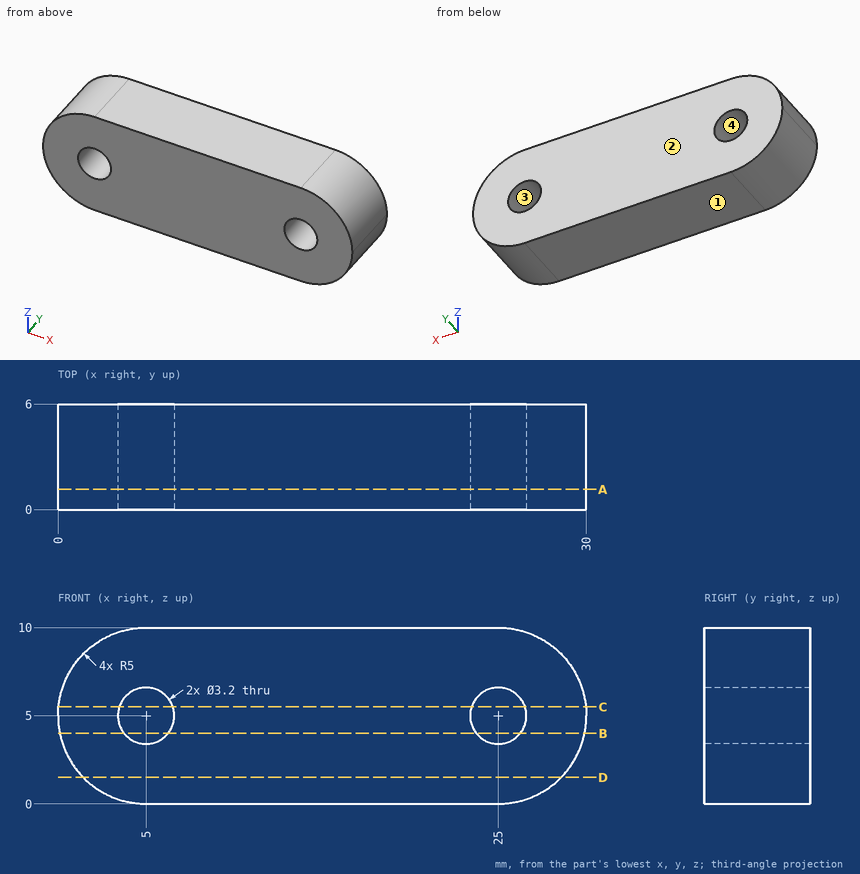
Design review of the part shown in the three views and the two pictorial views. Dimensions are in mm from the part's minimum x, y and z. Give positions to 0.01 mm unless a question says otherwise; leave off trailing zeros. Loops run counter-clockwise (first coordinate to the right, second up) from the corner with the lowest first, then second, coordinate; pieces in that order, holes last. Notation, with made-up numbers: (37.25, -12) -> (62.25, -12) arc R17 ccw to (62.25, 12) -> close; hole circle Ø7 at (48.5, 9). An arc over 180 degrees is marked (long way). One line per question, with ' | ' between items.
1) We need section A-A (y = 1.15). Give the number of separate pieces and of enclosed holes in the cut face, plus the area to 3 significant figures.
Resolved:
separate pieces: 1 | enclosed holes: 2 | area: 262 mm2
2) We need section D-D (z = 1.5). Write out the cut boundary in (x, y), plus the area to 3 significant figures.
Resolved:
outline: (1.43, 0) -> (28.57, 0) -> (28.57, 6) -> (1.43, 6) -> close | area: 163 mm2
3) We need section C-C (z = 5.5). Write out the cut boundary in (x, y) (3 decimals), plus the area to 3 significant figures.
Resolved:
outline: (0.025, 0) -> (3.48, 0) -> (3.48, 6) -> (0.025, 6) -> close; (6.52, 0) -> (23.48, 0) -> (23.48, 6) -> (6.52, 6) -> close; (26.52, 0) -> (29.975, 0) -> (29.975, 6) -> (26.52, 6) -> close | area: 143 mm2
4) Insertion check: pin 1 Ø2 at (y, z) = (5, 7) entering from +X. The pin has a flat end and moves straight along its axis. Give the tip position at first contact, or say it passes through.
Resolved:
pin 1: stops at x = 29.9
5) The part is to be moulded in two halves that separate along Z. For the marked faces 1, 2, 3 and 4, say which applies: +Z half, -Z half, draft (parallel to the pull), parting line (faces both ways), or undercut.
Resolved:
face 1: -Z half | face 2: draft | face 3: undercut | face 4: undercut
6) To check wall thickness, follow probe 1 along Z at (x, y) = (25, 1.5); probe 2 along X at (y, z) = (4.8, 4.5) (3 decimals); probe 3 along X at (y, z) = (1.15, 3.75). State the ranges of each line that lie inside material, in increasing order.
Resolved:
probe 1: z = 0 to 3.4, 6.6 to 10 | probe 2: x = 0.025 to 3.48, 6.52 to 23.48, 26.52 to 29.975 | probe 3: x = 0.16 to 4, 6 to 24, 26 to 29.84
7) We need section B-B (z = 4). Write out the cut boundary in (x, y), plus the area to 3 significant figures.
Resolved:
outline: (0.1, 0) -> (3.75, 0) -> (3.75, 6) -> (0.1, 6) -> close; (6.25, 0) -> (23.75, 0) -> (23.75, 6) -> (6.25, 6) -> close; (26.25, 0) -> (29.9, 0) -> (29.9, 6) -> (26.25, 6) -> close | area: 149 mm2
